Work out the finished part from the listing and answer in its coordinate system (mm). Round coordinates to 2 decimals unless told otherwise and drop trailing zeros. Loops run counter-clockwise (first coordinate to the right, second up) from the corner with the lowest first, then second, coordinate; pieces in that order, holes last. Notation, with made-up numbers: (82, -19) - (139, -19) arc R14 ccw to (139, -14) - close; hole circle Ø9 at (66.5, 9.25). An arc over 180 degrees is marked (long way). Return JSON: item names as keys, results as strings.
from build123d import *

# Parameters (mm, degrees)
BOSS_EXTRUDE1_DEPTH = 7.9375
BOSS_EXTRUDE4_DEPTH = 89.2175
CUT_EXTRUDE2_DEPTH  = 98.63800417


with BuildPart() as part:
    # Sketch2 → Boss-Extrude1 (new body)
    with BuildSketch(Plane.XY):
        Polygon((7.332348419, 0), (3.666174209, 6.35), (-3.666174209, 6.35), (-7.332348419, 0), (-3.666174209, -6.35), (3.666174209, -6.35), align=None)
    extrude(amount=BOSS_EXTRUDE1_DEPTH)

    # Sketch5 → Boss-Extrude4 (add)
    with BuildSketch(Plane.XY.offset(7.9375)):
        Polygon((7.332348419, 0), (3.666174209, 6.35), (-3.666174209, 6.35), (-7.332348419, 0), (-3.666174209, -6.35), (3.666174209, -6.35), align=None)
    extrude(amount=BOSS_EXTRUDE4_DEPTH)

    # Sketch6 → Cut-Extrude2 (cut, through all)
    with BuildSketch(Plane.XY.offset(97.155)):
        with BuildLine():
            ThreePointArc((-4.181770802, 5.456960506), (-3.4375, 5.953924651), (-2.634981025, 6.35))
            Line((-2.634981025, 6.35), (-3.666174209, 6.35))
            Line((-3.666174209, 6.35), (-4.181770802, 5.456960506))
        make_face()
        with BuildLine():
            ThreePointArc((2.634981025, 6.35), (3.4375, 5.953924651), (4.181770802, 5.456960506))
            Line((4.181770802, 5.456960506), (3.666174209, 6.35))
            Line((3.666174209, 6.35), (2.634981025, 6.35))
        make_face()
        with BuildLine():
            ThreePointArc((6.816751826, 0.893039494), (6.875, 0), (6.816751826, -0.893039494))
            Line((6.816751826, -0.893039494), (7.332348419, 0))
            Line((7.332348419, 0), (6.816751826, 0.893039494))
        make_face()
        with BuildLine():
            Line((2.634981025, -6.35), (3.666174209, -6.35))
            Line((3.666174209, -6.35), (4.181770802, -5.456960506))
            ThreePointArc((4.181770802, -5.456960506), (3.4375, -5.953924651), (2.634981025, -6.35))
        make_face()
        with BuildLine():
            Line((-3.666174209, -6.35), (-2.634981025, -6.35))
            ThreePointArc((-2.634981025, -6.35), (-3.4375, -5.953924651), (-4.181770802, -5.456960506))
            Line((-4.181770802, -5.456960506), (-3.666174209, -6.35))
        make_face()
        with BuildLine():
            Line((-7.332348419, 0), (-6.816751826, -0.893039494))
            ThreePointArc((-6.816751826, -0.893039494), (-6.875, 0), (-6.816751826, 0.893039494))
            Line((-6.816751826, 0.893039494), (-7.332348419, 0))
        make_face()
    extrude(amount=-CUT_EXTRUDE2_DEPTH, mode=Mode.SUBTRACT)


solid = part.part
1) Section C-C (x = 6) is taken. Give the vertices of the cut face in (y, z) (3 decimals), and give its area (3 significant figures).
Verdict:
{"outline": "(-2.308, 0) - (2.308, 0) - (2.308, 97.155) - (-2.308, 97.155) - close", "area": "448 mm2"}
2) Section A-A (z = 32) is taken. Give the vertices of the cut face in (x, y) (3 decimals).
Verdict:
{"outline": "(-6.817, -0.893) - (-4.182, -5.457) arc R6.875 ccw to (-2.635, -6.35) - (2.635, -6.35) arc R6.875 ccw to (4.182, -5.457) - (6.817, -0.893) arc R6.875 ccw to (6.817, 0.893) - (4.182, 5.457) arc R6.875 ccw to (2.635, 6.35) - (-2.635, 6.35) arc R6.875 ccw to (-4.182, 5.457) - (-6.817, 0.893) arc R6.875 ccw to start"}
3) Find the intervals of material crossed by L1, parallel to X at y = 2, z = 41.5; L2, parallel to X at y = -3, z = 66; L3, parallel to Y at x = -6, z = 28, in increasing order.
Verdict:
{"L1": "x = -6.18 to 6.18", "L2": "x = -5.6 to 5.6", "L3": "y = -2.31 to 2.31"}
4) Flat-ended cylindrical pins translate along their axes: pin 1 (2 mm diameter, centred on y = 3, z = 66.5, fed in from -X); pin 2 (5 mm diameter, centred on y = 4.5, z = 51, fed in from +X). Find the tip coordinate at first contact, or state that the pin passes through.
Verdict:
{"pin 1": "stops at x = -6.18", "pin 2": "stops at x = 6.18"}
5) Section B-B (y = -1.75) is taken. Give the vertices of the cut face in (x, z) (3 decimals), and give its area (3 significant figures).
Verdict:
{"outline": "(-6.322, 0) - (6.322, 0) - (6.322, 97.155) - (-6.322, 97.155) - close", "area": "1,230 mm2"}
